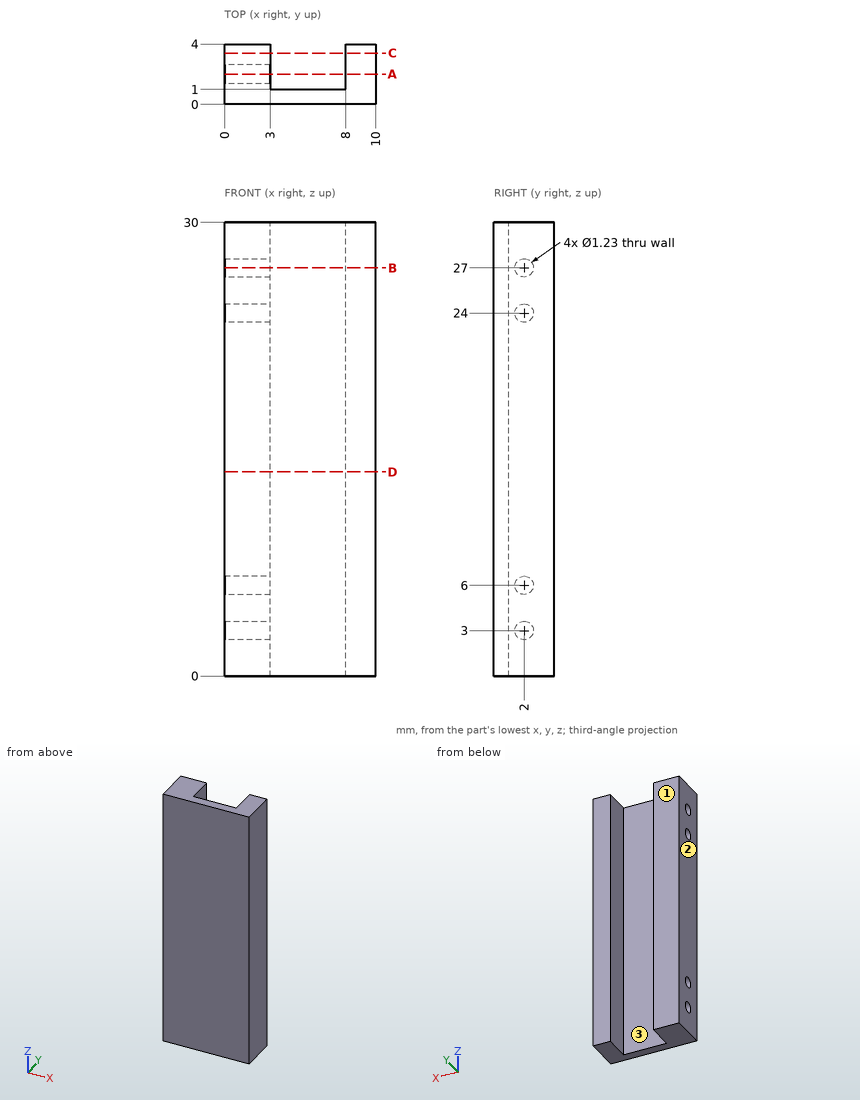
Here's the drawing with two shaded views (mm, measured from the low corner). I have some questions. Give positions to 0.01 mm unless a question says otherwise; leave off trailing zeros. Write each loop counter-clockwise with the first axis right and the second up, starting at its lowest first coordinate (ties: lowest second). Pieces come first, ordered by that corner, then holes. Notation, with made-up numbers: (44, -29) -> (50, -29) arc R29 ccw to (50, 1) -> close; hole circle Ø1 at (84, 60.25). An arc over 180 degrees is marked (long way). Answer as a JSON object with one key per item and string values. Group by question number.
Item 1: Suppose I cut it at B-B (z = 27). Please give me the cut outline in (x, y) (3 decimals), plus the area to 3 significant figures.
Item 2: Please list where these lines run through material, in increasing order: line 1 (X direction, y = 2.6, z = 3.5); line 2 (Y direction, x = 2.45, z = 27) (3 decimals); line 3 (Z direction, x = 1.5, y = 2.35). Write a range as [from, to].
Item 3: Suppose I cut it at C-C (y = 3.4). Please give me the cut outline in (x, z).
Item 4: Suppose I cut it at D-D (z = 13.5). Please give me the cut outline in (x, y).
Item 5: Suppose I cut it at A-A (y = 2). Please give me the cut outline in (x, z) (3 decimals), plus the area to 3 significant figures.
Item 6: We'd pull the mould along X, two halves only. Please class the marked faces 1, 2 and 3: +X half, -X half, draft (parallel to the pull), parting line (faces both ways), or undercut.
Item 7: I'm going to push a flat-ended pin straight in: P1, Ø2.5, axis at x = 6.5, z = 20.5, coming from the +Y side. Where does the tip first touch, or does it pass through?
Findings:
{
 "1": {"outline": "(0, 0) -> (10, 0) -> (10, 4) -> (8, 4) -> (8, 1) -> (3, 1) -> (3, 1.385) -> (0, 1.385) -> close; (0, 2.615) -> (3, 2.615) -> (3, 4) -> (0, 4) -> close", "area": "21.3 mm²"},
 "2": {"line 1": "x = [0, 3], [8, 10]", "line 2": "y = [0, 1.385], [2.615, 4]", "line 3": "z = [0, 2.49], [3.51, 5.49], [6.51, 23.49], [24.51, 26.49], [27.51, 30]"},
 "3": {"outline": "(0, 0) -> (3, 0) -> (3, 30) -> (0, 30) -> close; (8, 0) -> (10, 0) -> (10, 30) -> (8, 30) -> close"},
 "4": {"outline": "(0, 0) -> (10, 0) -> (10, 4) -> (8, 4) -> (8, 1) -> (3, 1) -> (3, 4) -> (0, 4) -> close"},
 "5": {"outline": "(0, 0) -> (3, 0) -> (3, 2.385) -> (0, 2.385) -> close; (0, 3.615) -> (3, 3.615) -> (3, 5.385) -> (0, 5.385) -> close; (0, 6.615) -> (3, 6.615) -> (3, 23.385) -> (0, 23.385) -> close; (0, 24.615) -> (3, 24.615) -> (3, 26.385) -> (0, 26.385) -> close; (0, 27.615) -> (3, 27.615) -> (3, 30) -> (0, 30) -> close; (8, 0) -> (10, 0) -> (10, 30) -> (8, 30) -> close", "area": "135 mm²"},
 "6": {"face 1": "draft", "face 2": "-X half", "face 3": "undercut"},
 "7": {"P1": "stops at y = 1"}
}
